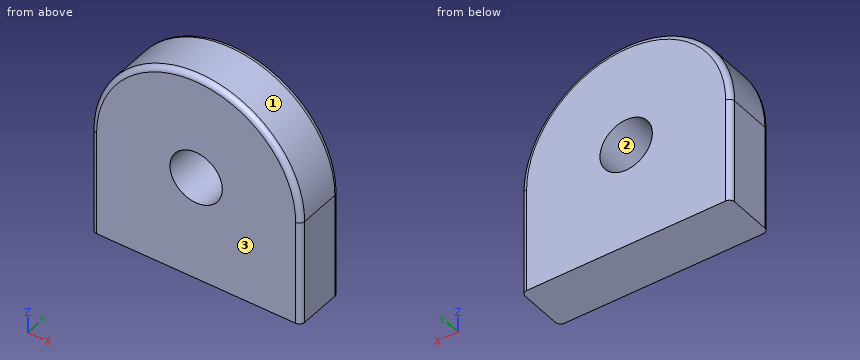
from build123d import *

# Parameters (mm, degrees)
F0_R     = 2.5
F1_DEPTH = 5
F2_R     = 0.5


with BuildPart() as f1:
    # F0 (on Front) → F1 (new body)
    with BuildSketch(Plane.XZ):
        with BuildLine():
            Line((-10, 12.10352), (10, 12.10352))
            Line((10, 12.10352), (10, 22.10352))
            ThreePointArc((10, 22.10352), (0, 32.10352), (-10, 22.10352))
            Line((-10, 22.10352), (-10, 12.10352))
        make_face()
        with Locations((0, 22.10352)):
            Circle(F0_R, mode=Mode.SUBTRACT)
    extrude(amount=F1_DEPTH)

    # F2
    f2_edges = [f1.edges().sort_by_distance(p)[0] for p in [
        (0, -5, 32.10352),
        (10, 0, 17.10352),
    ]]
    fillet(f2_edges, radius=F2_R)


solid = f1.part
Geometry check sheet. Reference: the model listing, model coordinates, mm. Face numbers are marked on the shaded views. Coordinates: 2 decimals unless noted, no trailing zeros. Order: outer loops, then holes, each group sorted by start corner. A loop starts at its lowest first (then second) coordinate and runs counter-clockwise, first axis right, second up. Notation, with made-up numbers: (-4.75, 74.5) -> (37.25, 74.5) arc R21 ccw to (37.25, 80.5) -> close; hole circle Ø5 at (31, 79.25). An arc over 180 degrees is marked (long way). Use a Markdown table: item, result. Add a question column.
1. Cross-section at B-B (y = -1.85). Enter the section's corners in (x, z), and give its area (3 significant figures).
2. Material ranges on L1, parallel to Z at x = 0, y = -3.8; L2, parallel to X at y = -0.75, z = 23; L3, parallel to X at y = -1.15, z = 20.75, recorded low to high.
3. Cross-section at A-A (x = 0). Enter the section's corners in (y, z).
4. Mould release check, pull along Z, two halves, no side actions. Record for the marked faces 1, 2 and 3: pulls with the +Z half, pulls with the -Z half, needs draft (parallel to the pull), parting line crosses it, or undercut.
5. Go/stop test with flat-tipped pins: pin 1 Ø1.5 at (x, y) = (3, -1.5) entering from +Z; pin 2 Ø1 at (y, z) = (-1, 25.5) entering from +X. Record where each tip stops, or that it passes through.
6. Cross-section at C-C (z = 21.5). Enter the section's corners in (x, y), and give its area (3 significant figures).
Filled sheet:
| question | item | result |
|---|---|---|
| 1 | outline | (-10, 12.1) -> (10, 12.1) -> (10, 22.1) arc R10 ccw to (-10, 22.1) -> close; hole circle Ø5 at (0, 22.1) |
| 1 | area | 337 mm2 |
| 2 | L1 | 12.1 to 19.6, 24.6 to 32.1 |
| 2 | L2 | -9.96 to -2.33, 2.33 to 9.96 |
| 2 | L3 | -10 to -2.1, 2.1 to 10 |
| 3 | outline | (-5, 12.1) -> (0, 12.1) -> (0, 19.6) -> (-5, 19.6) -> close; (-5, 24.6) -> (0, 24.6) -> (0, 31.6) arc R0.5 ccw to (-0.5, 32.1) -> (-4.5, 32.1) arc R0.5 ccw to (-5, 31.6) -> close |
| 4 | face 1 | pulls with the +Z half |
| 4 | face 2 | undercut |
| 4 | face 3 | needs draft |
| 5 | pin 1 | z = 31.85 |
| 5 | pin 2 | x = 9.57 |
| 6 | outline | (-10, -4.5) arc R0.5 ccw to (-9.5, -5) -> (-2.43, -5) -> (-2.43, 0) -> (-9.5, 0) arc R0.5 ccw to (-10, -0.5) -> close; (2.43, -5) -> (9.5, -5) arc R0.5 ccw to (10, -4.5) -> (10, -0.5) arc R0.5 ccw to (9.5, 0) -> (2.43, 0) -> close |
| 6 | area | 75.5 mm2 |
